For this review, take the finished solid that the model builds, in its own axes (mm). A direction names the side the tool comes from. Round coordinates to 2 decimals unless told otherwise and drop trailing zeros. Answer in a Markdown table with one row per item.
from build123d import *

# Parameters (mm, degrees)
SKETCH1_R           = 2.1
BOSS_EXTRUDE1_DEPTH = 340
EXTRUDE_1_DEPTH     = 20


with BuildPart() as part:
    # Sketch1 → Boss-Extrude1 (new body)
    with BuildSketch(Plane.XY):
        Polygon((-10, 10), (-10, 5), (-8.2, 3.2), (-8.2, 5.499339828), (-6.56, 5.499339828), (-3.900660172, 2.84), (-3.900660172, -2.84), (-6.56, -5.499339828), (-8.2, -5.499339828), (-8.2, -3.2), (-10, -5), (-10, -10), (-5, -10), (-3.2, -8.2), (-5.499339828, -8.2), (-5.499339828, -6.56), (-2.84, -3.900660172), (2.84, -3.900660172), (5.499339828, -6.56), (5.499339828, -8.2), (3.2, -8.2), (5, -10), (10, -10), (10, -5), (8.2, -3.2), (8.2, -5.499339828), (6.56, -5.499339828), (3.900660172, -2.84), (3.900660172, 2.84), (6.56, 5.499339828), (8.2, 5.499339828), (8.2, 3.2), (10, 5), (10, 10), (5, 10), (3.2, 8.2), (5.499339828, 8.2), (5.499339828, 6.56), (2.84, 3.900660172), (-2.84, 3.900660172), (-5.499339828, 6.56), (-5.499339828, 8.2), (-3.2, 8.2), (-5, 10), align=None)
        Circle(SKETCH1_R, mode=Mode.SUBTRACT)
    extrude(amount=-BOSS_EXTRUDE1_DEPTH)

    # 草图1 → 凸台-拉伸1 (add)
    with BuildSketch(Plane.XY):
        Polygon((-5, 10), (-10, 10), (-10, 5), (-8.2, 3.2), (-8.2, 5.499339828), (-6.56, 5.499339828), (-3.900660172, 2.84), (-3.900660172, -2.84), (-6.56, -5.499339828), (-8.2, -5.499339828), (-8.2, -3.2), (-10, -5), (-10, -10), (-5, -10), (-3.2, -8.2), (-5.499339828, -8.2), (-5.499339828, -6.56), (-2.84, -3.900660172), (2.84, -3.900660172), (5.499339828, -6.56), (5.499339828, -8.2), (3.2, -8.2), (5, -10), (10, -10), (10, -5), (8.2, -3.2), (8.2, -5.499339828), (6.56, -5.499339828), (3.900660172, -2.84), (3.900660172, 2.84), (6.56, 5.499339828), (8.2, 5.499339828), (8.2, 3.2), (10, 5), (10, 10), (5, 10), (3.2, 8.2), (5.499339828, 8.2), (5.499339828, 6.56), (2.84, 3.900660172), (-2.84, 3.900660172), (-5.499339828, 6.56), (-5.499339828, 8.2), (-3.2, 8.2), align=None)
    extrude(amount=EXTRUDE_1_DEPTH)


solid = part.part
1) Clearance check with flat-ended pins moving along their axes: pin 1 Ø0.7 at (x, z) = (-4.5, -173.5) entering from +Y; pin 2 Ø1.1 at (y, z) = (-4, -201) entering from -X; pin 3 Ø5 at (x, z) = (2, -51.5) entering from -Y. State where each tip first meets the part, or that it passes through.
Solved:
| item | result |
|---|---|
| pin 1 | y = 9.85 |
| pin 2 | x = -9.55 |
| pin 3 | y = -9.5 |
2) For faces 1 (the flat face through (0, 0, 20)), 2 (the flat face through (3.901, 0, -163)), 3 (the flat face through (0, -3.901, -163)), list the 3-axis set-ups (+Z, -Z, +X, -X, +Y, -Y) from which the entire face can be reached by the end or side of a thin tool; tool diameter is ignored.
Solved:
| item | result |
|---|---|
| face 1 | +Z, +X, -X, +Y, -Y |
| face 2 | +Z, -Z, +X |
| face 3 | +Z, -Z, -Y |
3) Mouldability with a two-part tool opening along Y and no side actions: class faces 4 (the flat face through (-2.4, 0.1, -340)), 5 (the flat face through (-3.901, 0, -163)), 6 (the flat face through (0, 3.901, -163)) as pulls with the +Y half, pulls with the -Y half, needs draft (parallel to the pull), parting line crosses it, or undercut.
Solved:
| item | result |
|---|---|
| face 4 | needs draft |
| face 5 | undercut |
| face 6 | pulls with the +Y half |
4) For line 1 (Y direction, x = -7, z = -305); line 2 (Y direction, x = -0.25, z = -176.5); line 3 (X direction, y = -4, z = -309.5), list the stretches that pass through material, from the lowest coordinate up. Write a range as [from, to].
Solved:
| item | result |
|---|---|
| line 1 | [-10, -5.5], [5.5, 10] |
| line 2 | [-3.9, -2.09], [2.09, 3.9] |
| line 3 | [-9, -8.2], [-5.06, -2.94], [2.94, 5.06], [8.2, 9] |
